Autodesk Inventor part; units mm, degrees
ref_plane "YZ Plane" through (0, 0, 0) normal (1, 0, 0) x (0, 1, 0)
ref_plane "XZ Plane" through (0, 0, 0) normal (0, 1, 0) x (-1, 0, 0)
ref_plane "XY Plane" through (0, 0, 0) normal (0, 0, 1) x (1, 0, 0)
sketch "Skizze1" plane through (0, 0, 0) normal (0, 1, 0) x (-1, 0, 0)
  line L0 (0, 18) -> (3, 18)
  line L1 (3, 18) -> (3, 12)
  line L2 (3, 12) -> (4.5, 12)
  line L3 (4.5, 12) -> (4.5, -12)
  line L4 (4.5, -12) -> (3, -12)
  line L5 (3, -12) -> (3, -18)
  line L6 (3, -18) -> (0, -18)
  line L7 (0, -18) -> (0, 18)
  point P0 (0, 0)
  point P1 (0, 0)
  dimension "d0" = 6
  dimension "d1" = 6
  dimension "d2" = 24
  dimension "d3" = 9
  dimension "d4" = 6
revolve "Umdrehung1" add sketch "Skizze1" angle 360 about axis through (0, 0, -18) along (0, 0, 1)
thread "Gewinde1"
thread "Gewinde2"
properties part number "welle_verbindung"
The model under review builds one solid part; all positions refer to its coordinate system, in mm. A direction names the side the tool comes from. Round coordinates to 2 decimals unless told otherwise and drop trailing zeros. Loops run counter-clockwise (first coordinate to the right, second up) from the corner with the lowest first, then second, coordinate; pieces in that order, holes last.
1) Clearance check with flat-ended pins moving along their axes: P1, Ø4, axis at y = -2.5, z = 10, coming from the +X side; P2, Ø1, axis at y = -2, z = 9.5, coming from the -X side; P3, Ø1.5, axis at x = 3, z = -7.5, coming from the +Y side. State where each tip first meets the part, or that it passes through.
Values follow:
P1: stops at x = 4.47
P2: stops at x = -4.24
P3: stops at y = 3.9
2) Wall thickness on line 1 along Y through (x, z) = (-0.25, -9.5); line 2 along Z through (x, y) = (-1.25, 4); line 3 along Y through (x, z) = (-2.25, -14): over which ranges is each line inside the solid? List them lowest first.
Values follow:
line 1: y = -4.49 to 4.49
line 2: z = -12 to 12
line 3: y = -1.98 to 1.98
3) Consider section B-B on x = -0.75. State the section outline as (y, z) points.
Values follow:
outline: (-4.44, -12) - (-2.9, -12) - (-2.9, -18) - (2.9, -18) - (2.9, -12) - (4.44, -12) - (4.44, 12) - (2.9, 12) - (2.9, 18) - (-2.9, 18) - (-2.9, 12) - (-4.44, 12) - close
4) Consider section A-A on y = 0. State the section outline as (x, z) points.
Values follow:
outline: (-4.5, -12) - (-3, -12) - (-3, -18) - (3, -18) - (3, -12) - (4.5, -12) - (4.5, 12) - (3, 12) - (3, 18) - (-3, 18) - (-3, 12) - (-4.5, 12) - close
5) Consider section C-C on z = 1. State the section outline as (x, y) points, then the cut area to 3 significant figures.
Values follow:
outline: circle Ø9 at (0, 0)
area: 63.6 mm2
6) Tool access review of faces 1 (the face through (-1, 3, 12)), 2 (the face through (3, 0, -15)), 3 (the face through (0, 0, -18)): name each direction out of +Z, -Z, +X, -X, +Y, -Y from which nothing blocks a thin tool from reaching the whole face with its end or side.
Values follow:
face 1: +Z
face 2: -Z
face 3: -Z, +X, -X, +Y, -Y
